from build123d import *

# Parameters (mm, degrees)
F0_W     = 85.09
F0_H     = 95.25
F1_DEPTH = 6.35
F2_R     = 1.905
F3_DEPTH = 6.351


with BuildPart() as f1:
    # F0 (on Top) → F1 (new body)
    with BuildSketch(Plane.XY):
        Rectangle(F0_W, F0_H)
    extrude(amount=F1_DEPTH)

    # F2 (on Top) → F3 (cut, through all)
    with BuildSketch(Plane.XY):
        with Locations((-32.22625, -35.983333)):
            Circle(F2_R)
        with Locations((-32.22625, -12.691533)):
            Circle(F2_R)
        with Locations((-32.22625, 10.600267)):
            Circle(F2_R)
        with Locations((-32.22625, 33.892067)):
            Circle(F2_R)
        with Locations((-32.22625, 57.183867)):
            Circle(F2_R)
        with Locations((-32.22625, 80.475667)):
            Circle(F2_R)
        with Locations((-11.60145, -35.983333)):
            Circle(F2_R)
        with Locations((-11.60145, -12.691533)):
            Circle(F2_R)
        with Locations((-11.60145, 10.600267)):
            Circle(F2_R)
        with Locations((-11.60145, 33.892067)):
            Circle(F2_R)
        with Locations((-11.60145, 57.183867)):
            Circle(F2_R)
        with Locations((-11.60145, 80.475667)):
            Circle(F2_R)
        with Locations((9.02335, -35.983333)):
            Circle(F2_R)
        with Locations((9.02335, -12.691533)):
            Circle(F2_R)
        with Locations((9.02335, 10.600267)):
            Circle(F2_R)
        with Locations((9.02335, 33.892067)):
            Circle(F2_R)
        with Locations((9.02335, 57.183867)):
            Circle(F2_R)
        with Locations((9.02335, 80.475667)):
            Circle(F2_R)
        with Locations((29.64815, -35.983333)):
            Circle(F2_R)
        with Locations((29.64815, -12.691533)):
            Circle(F2_R)
        with Locations((29.64815, 10.600267)):
            Circle(F2_R)
        with Locations((29.64815, 33.892067)):
            Circle(F2_R)
        with Locations((29.64815, 57.183867)):
            Circle(F2_R)
        with Locations((29.64815, 80.475667)):
            Circle(F2_R)
    extrude(amount=F3_DEPTH, mode=Mode.SUBTRACT)


solid = f1.part
Work out the finished part from the listing and answer in its coordinate system (mm). Give positions to 0.01 mm unless a question says otherwise; leave off trailing zeros. Order: outer loops, then holes, each group sorted by start corner. A loop starts at its lowest first (then second) coordinate and runs counter-clockwise, first axis right, second up. Notation, with made-up numbers: (11.5, 34) - (59.5, 34) arc R10 cw to (59.5, 47) - close; hole circle Ø7 at (20, 3.25). An arc over 180 degrees is marked (long way). Answer as CSV lines item,"result". Start each with the question number.
Q1. Find the intervals of material crossed by L1, parallel to X at y = -12.5, z = 1.5 (1 decimal); L2, parallel to Y at x = -10.5, z = 2.25 (3 decimals); L3, parallel to X at y = -35, z = 3.5 (3 decimals), in increasing order. Write a range as [from, to].
Q2. The part is cut by section B-B (z = 3). Give the number of separate pieces and of enclosed holes in the cut face, then the cut area to 3 significant figures.
Q3. Given pin 1 Ø6 at (x, y) = (29.65, 10.6) entering from +Z, flat-ended and moving along its own axis, determine where the tip first touches the part or whether it passes through.
Q4. The mould has two halves that part along Y. Classify faces 1 (the face through (-1, -47.625, 3)), 2 (the face through (-32.639, 32.032, 3.131)), 3 (the face through (30.672, -34.377, 3.131)), 4 (the face through (-1, 1, 0)): +Y half, -Y half, draft (parallel to the pull), parting line (faces both ways), or undercut.
Q5. The part is cut by section A-A (x = -32). Write down the section's boundary in (y, z) (3 decimals).
Check result:
1,L1,"x = [-42.5, -34.1], [-30.3, -13.5], [-9.7, 7.1], [10.9, 27.8], [31.5, 42.5]"
1,L2,"y = [-47.625, -37.538], [-34.429, -14.246], [-11.137, 9.046], [12.155, 32.338], [35.446, 47.625]"
1,L3,"x = [-42.545, -33.858], [-30.595, -13.233], [-9.97, 7.392], [10.655, 28.017], [31.28, 42.545]"
2,separate pieces,"1"
2,enclosed holes,"16"
2,area,"7,920 mm²"
3,pin 1,"stops at z = 6.35"
4,face 1,"-Y half"
4,face 2,"undercut"
4,face 3,"undercut"
4,face 4,"draft"
5,outline,"(-47.625, 0) - (-37.875, 0) - (-37.875, 6.35) - (-47.625, 6.35) - close; (-34.092, 0) - (-14.583, 0) - (-14.583, 6.35) - (-34.092, 6.35) - close; (-10.8, 0) - (8.709, 0) - (8.709, 6.35) - (-10.8, 6.35) - close; (12.492, 0) - (32.001, 0) - (32.001, 6.35) - (12.492, 6.35) - close; (35.784, 0) - (47.625, 0) - (47.625, 6.35) - (35.784, 6.35) - close"
